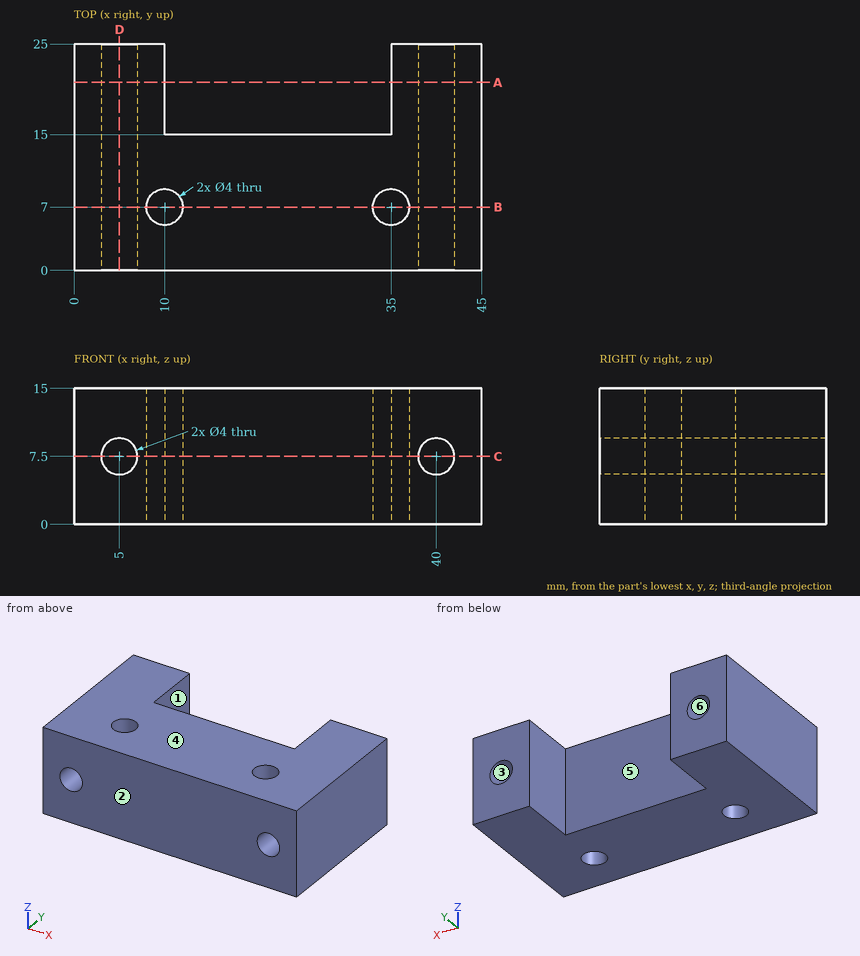
Part print with two shaded views. Sizes in mm from the minimum x, y, z corner. A direction names the side the tool comes from. Round coordinates to 2 decimals unless told otherwise and drop trailing zeros. Loops run counter-clockwise (first coordinate to the right, second up) from the corner with the lowest first, then second, coordinate; pieces in that order, holes last.
1. 3-axis set-ups, long thin cutter, end or side, ignore diameter. For the marked faces 1 and 2: which of +Z, -Z, +X, -X, +Y, -Y reach the whole face in a straight line?
Solutions:
face 1: +Z, -Z, +Y
face 2: +Z, -Z, +X, -X, -Y
2. Flat gauge pin, fed straight in: pin 1 (2.5 mm diameter, centred on x = 5, z = 7.5, fed in from -Y). Where does the tip first touch, or does it go through?
Solutions:
pin 1: passes through
3. Slice it at C-C (z = 7.5). Give the cut face in (x, y).
Solutions:
outline: (0, 0) - (3, 0) - (3, 25) - (0, 25) - close; (7, 0) - (38, 0) - (38, 25) - (35, 25) - (35, 15) - (10, 15) - (10, 25) - (7, 25) - close; (42, 0) - (45, 0) - (45, 25) - (42, 25) - close; hole circle Ø4 at (10, 7); hole circle Ø4 at (35, 7)
4. Slice it at B-B (y = 7). Give the cut face in (x, z), and give its area (3 significant figures).
Solutions:
outline: (0, 0) - (8, 0) - (8, 15) - (0, 15) - close; (12, 0) - (33, 0) - (33, 15) - (12, 15) - close; (37, 0) - (45, 0) - (45, 15) - (37, 15) - close; hole circle Ø4 at (5, 7.5); hole circle Ø4 at (40, 7.5)
area: 530 mm2
5. Drill centre lines: line 1 along X through (y, z) = (14.75, 7.5); line 2 along X through (y, z) = (19.5, 7.5); line 3 along X through (y, z) = (7, 5). Where is each one in solid material? Low to high.
Solutions:
line 1: x = 0 to 3, 7 to 38, 42 to 45
line 2: x = 0 to 3, 7 to 10, 35 to 38, 42 to 45
line 3: x = 0 to 8, 12 to 33, 37 to 45
6. Slice it at A-A (y = 20.75). Give the cut face in (x, z), and give its area (3 significant figures).
Solutions:
outline: (0, 0) - (10, 0) - (10, 15) - (0, 15) - close; (35, 0) - (45, 0) - (45, 15) - (35, 15) - close; hole circle Ø4 at (5, 7.5); hole circle Ø4 at (40, 7.5)
area: 275 mm2
7. Slice it at D-D (x = 5). Give the cut face in (y, z).
Solutions:
outline: (0, 0) - (25, 0) - (25, 5.5) - (0, 5.5) - close; (0, 9.5) - (25, 9.5) - (25, 15) - (0, 15) - close
8. Two-plate mould, pull along Z, no slides. Class the marked faces 3, 4, 5 and 6: pulls with the +Z half, pulls with the -Z half, needs draft (parallel to the pull), parting line crosses it, or undercut.
Solutions:
face 3: undercut
face 4: pulls with the +Z half
face 5: needs draft
face 6: undercut
